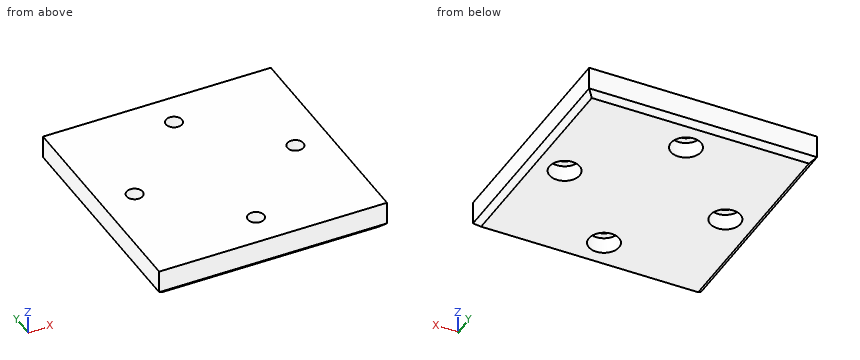
from build123d import *

# Parameters (mm, degrees)
F0_W     = 85
F0_H     = 85
F1_DEPTH = 10.5
F4_R     = 3
F5_DEPTH = 25
F6_R     = 5.65
F6_R_2   = 3
F7_DEPTH = 6
F8_SIZE  = 2


with BuildPart() as f1:
    # F0 (on Top) → F1 (new body)
    with BuildSketch(Plane.XY):
        Rectangle(F0_W, F0_H)
    extrude(amount=F1_DEPTH)

    # F4 (on face) → F5 (cut)
    with BuildSketch(Plane(origin=(0, 0, 0), x_dir=(1, 0, 0), z_dir=(0, 0, -1))):
        with Locations((0, 30)):
            Circle(F4_R)
        with Locations((0, -30)):
            Circle(F4_R)
        with Locations((30, 0)):
            Circle(F4_R)
        with Locations((-30, 0)):
            Circle(F4_R)
    extrude(amount=-F5_DEPTH, mode=Mode.SUBTRACT)

    # F6 (on face) → F7 (cut)
    with BuildSketch(Plane(origin=(0, 0, 0), x_dir=(1, 0, 0), z_dir=(0, 0, -1))):
        with Locations((0, 30)):
            Circle(F6_R)
        with Locations((0, 30)):
            Circle(F6_R_2, mode=Mode.SUBTRACT)
        with Locations((30, 0)):
            Circle(F6_R)
        with Locations((30, 0)):
            Circle(F6_R_2, mode=Mode.SUBTRACT)
        with Locations((0, -30)):
            Circle(F6_R)
        with Locations((0, -30)):
            Circle(F6_R_2, mode=Mode.SUBTRACT)
        with Locations((-30, 0)):
            Circle(F6_R)
        with Locations((-30, 0)):
            Circle(F6_R_2, mode=Mode.SUBTRACT)
    extrude(amount=-F7_DEPTH, mode=Mode.SUBTRACT)

    # F8
    f8_edges = [f1.edges().sort_by_distance(p)[0] for p in [
        (-42.5, 0, 0),
        (0, -42.5, 0),
        (42.5, 0, 0),
        (0, 42.5, 0),
    ]]
    chamfer(f8_edges, length=F8_SIZE)


solid = f1.part
Read the model definition and answer for the solid it produces. Units are mm, in the model's axes. Round coordinates to 2 decimals unless told otherwise and drop trailing zeros. Write each loop counter-clockwise with the first axis right and the second up, starting at its lowest first coordinate (ties: lowest second). Pieces come first, ordered by that corner, then holes.
1. The part is cut by section A-A, the plane x = 0. Determine the outline of the cut face in (y, z), then the cut area to 3 significant figures.
2. Straight lines are drawn through the part: L1, parallel to Y at x = 0, z = 3.8; L2, parallel to Y at x = 30, z = 3.7. For each, find the intervals that lie inside material, in ascending order.
3. The part is cut by section B-B, the plane y = 30. Determine the outline of the cut face in (x, z), then the cut area to 3 significant figures.
4. Given pin 1 Ø5.5 at (x, y) = (0, -31.5) entering from -Z; pin 2 Ø5 at (x, y) = (0, -30) entering from +Z, each flat-ended and moving along its own axis, determine where each tip first touches the part or whether it passes through.
Values:
1. outline: (-42.5, 2) - (-40.5, 0) - (-35.65, 0) - (-35.65, 6) - (-33, 6) - (-33, 10.5) - (-42.5, 10.5) - close; (-27, 6) - (-24.35, 6) - (-24.35, 0) - (24.35, 0) - (24.35, 6) - (27, 6) - (27, 10.5) - (-27, 10.5) - close; (33, 6) - (35.65, 6) - (35.65, 0) - (40.5, 0) - (42.5, 2) - (42.5, 10.5) - (33, 10.5) - close
1. area: 699 mm2
2. L1: y = -42.5 to -35.65, -24.35 to 24.35, 35.65 to 42.5
2. L2: y = -42.5 to -5.65, 5.65 to 42.5
3. outline: (-42.5, 2) - (-40.5, 0) - (-5.65, 0) - (-5.65, 6) - (-3, 6) - (-3, 10.5) - (-42.5, 10.5) - close; (3, 6) - (5.65, 6) - (5.65, 0) - (40.5, 0) - (42.5, 2) - (42.5, 10.5) - (3, 10.5) - close
3. area: 794 mm2
4. pin 1: stops at z = 6
4. pin 2: passes through
